from build123d import *

# Parameters (mm, degrees)
F1_DEPTH = 22.5
F3_DEPTH = 4.5


with BuildPart() as f1:
    # F0 (on Front) → F1 (new body, symmetric)
    with BuildSketch(Plane.XZ):
        with BuildLine():
            Line((-30, 0), (-15, 0))
            ThreePointArc((-15, 0), (0, 15), (15, 0))
            Line((15, 0), (30, 0))
            ThreePointArc((30, 0), (0, 30), (-30, 0))
        make_face()
        with BuildLine():
            ThreePointArc((15, 0), (13.416407865, -6.7082039325), (9, -12))
            Line((9, -12), (9, -28.6181760425))
            ThreePointArc((9, -28.6181760425), (24.1867732449, -17.7482393493), (30, 0))
            Line((30, 0), (15, 0))
        make_face()
        with BuildLine():
            Line((-9, -28.6181760425), (-9, -12))
            ThreePointArc((-9, -12), (-13.416407865, -6.7082039325), (-15, 0))
            Line((-15, 0), (-30, 0))
            ThreePointArc((-30, 0), (-24.1867732449, -17.7482393493), (-9, -28.6181760425))
        make_face()
        with BuildLine():
            Line((-9, -60), (-9, -28.6181760425))
            ThreePointArc((-9, -28.6181760425), (-24.1867732449, -17.7482393493), (-30, 0))
            Line((-30, 0), (-30, -60))
            Line((-30, -60), (-9, -60))
        make_face()
        with BuildLine():
            ThreePointArc((30, 0), (24.1867732449, -17.7482393493), (9, -28.6181760425))
            Line((9, -28.6181760425), (9, -60))
            Line((9, -60), (30, -60))
            Line((30, -60), (30, 0))
        make_face()
    extrude(amount=F1_DEPTH, both=True)

    # F2 (on Front) → F3 (join, symmetric)
    with BuildSketch(Plane.XZ):
        with BuildLine():
            Line((-30, 90), (-30, 0))
            ThreePointArc((-30, 0), (0, 30), (30, 0))
            Line((30, 0), (30, 51))
            Line((30, 51), (0, 51))
            ThreePointArc((0, 51), (-9, 60), (0, 69))
            Line((0, 69), (30, 69))
            Line((30, 69), (30, 90))
            Line((30, 90), (-30, 90))
        make_face()
    extrude(amount=F3_DEPTH, both=True)


solid = f1.part
Model file for the job. Use its own axes, mm. A direction names the side the tool comes from. Give positions to 0.01 mm unless a question says otherwise; leave off trailing zeros. Order: outer loops, then holes, each group sorted by start corner. A loop starts at its lowest first (then second) coordinate and runs counter-clockwise, first axis right, second up. Notation, with made-up numbers: (63.5, 72) - (86.5, 72) arc R17 cw to (86.5, 102) - close; hole circle Ø9 at (-38, 62.25). An arc over 180 degrees is marked (long way). Write item = value, one per line. Start each with the question number.
1. Probe line 1 along X through (y, z) = (-18.5, -36.5); line 2 along Z through (x, y) = (0, 8); line 3 along Z through (x, y) = (11.5, -1). List the from-to ranges inside material, lowest first.
2. Two-plate mould, pull along X, no slides. Class faces 1 (the flat face through (-9, 0, -36)), 2 (the flat face through (-7, -4.5, 66)), 3 (the cylindrical face through (0.66, -13.626, 29.993)): pulls with the +X half, pulls with the -X half, needs draft (parallel to the pull), parting line crosses it, or undercut.
3. Cut at C-C, the plane x = -18. List the corners of the cut face in (y, z), and give its area (3 significant figures).
4. Cut at B-B, the plane y = 15. List the corners of the cut face in (x, z), and give its area (3 significant figures).
5. Cut at A-A, the plane x = 24. List the corners of the cut face in (y, z), and give its area (3 significant figures).
6. Cut at D-D, the plane z = 60. List the corners of the cut face in (x, y), and give its area (3 significant figures).
7. Drop flat-ended pins along their axis: P1, Ø4, axis at y = -16.5, z = 2.5, coming from the -X side; P2, Ø18, axis at x = 8, z = 63.5, coming from the -Y side; P3, Ø12, axis at x = -21, y = -14.5, coming from the +Z side. Give the stop position or say it passes through.
8. Which spindle directions (+Z, -Z, +X, -X, +Y, -Y) get a long thin tool onto all of the face, cutting with end or side? Do faces 4 (the flat face through (9, 0, -36)), 5 (the flat face through (-14, -22.5, -14)), 6 (the cylindrical face through (0.66, 13.374, 29.993)), 7 (the flat face through (15, 0, 69)). Say none if no direction does.
Taken from the geometry:
q1.line_1 = -30 to -9, 9 to 30
q1.line_2 = 15 to 30
q1.line_3 = -60 to -9.63, 9.63 to 51, 69 to 90
q2.face_1 = undercut
q2.face_2 = needs draft
q2.face_3 = parting line crosses it
q3.outline = (-22.5, -60) - (22.5, -60) - (22.5, 24) - (4.5, 24) - (4.5, 90) - (-4.5, 90) - (-4.5, 24) - (-22.5, 24) - close
q3.area = 4,370 mm²
q4.outline = (-30, -60) - (-9, -60) - (-9, -12) arc R15 cw (long way) to (9, -12) - (9, -60) - (30, -60) - (30, 0) arc R30 ccw to (-30, 0) - close
q4.area = 3,480 mm²
q5.outline = (-22.5, -60) - (22.5, -60) - (22.5, 18) - (4.5, 18) - (4.5, 51) - (-4.5, 51) - (-4.5, 18) - (-22.5, 18) - close; (-4.5, 69) - (4.5, 69) - (4.5, 90) - (-4.5, 90) - close
q5.area = 4,000 mm²
q6.outline = (-30, -4.5) - (-9, -4.5) - (-9, 4.5) - (-30, 4.5) - close
q6.area = 189 mm²
q7.P1 = -30
q7.P2 = -4.5
q7.P3 = 25.98
q8.face_4 = -Z, +Y, -Y
q8.face_5 = +Z, -Z, +X, -X, -Y
q8.face_6 = +Z, +Y
q8.face_7 = +X, +Y, -Y
